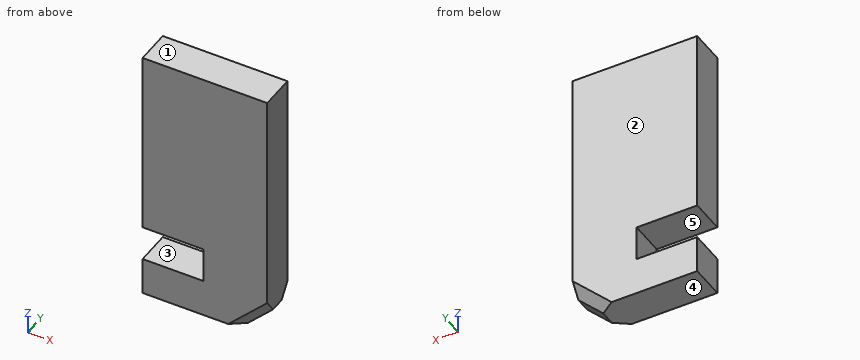
from build123d import *

# Parameters (mm, degrees)
EXTRUDE_1_DEPTH = 14
CHAMFER_1_SIZE  = 4


with BuildPart() as part:
    # 草图1 → 凸台-拉伸1 (new body)
    with BuildSketch(Plane(origin=(0, 0, 0), x_dir=(1, 0, 0), z_dir=(0, 1, 0))):
        Polygon((40, 105), (50, 95), (50, 0), (0, 0), (0, 75.675047551), (24.325372692, 75.675047551), (24.325372692, 89.813954871), (0, 89.813954871), (0, 105), align=None)
    extrude(amount=EXTRUDE_1_DEPTH)

    # 倒角1
    chamfer_1_edges = [part.edges().sort_by_distance(p)[0] for p in [
        (45, 0, -100),
        (45, 14, -100),
    ]]
    chamfer(chamfer_1_edges, length=CHAMFER_1_SIZE)


solid = part.part
Check sheet for the modelled part. Datum: model origin and axes. Units: mm. Face numbers are marked on the shaded views. A direction names the side the tool comes from. Give positions to 0.01 mm unless a question says otherwise; leave off trailing zeros. Order: outer loops, then holes, each group sorted by start corner. A loop starts at its lowest first (then second) coordinate and runs counter-clockwise, first axis right, second up. Notation, with made-up numbers: M 15.5,-40 L 24.5,-40 A24 ccw 24.5,-11 Z; hole C 15.5,88.5 d4. An arc over 180 degrees is marked long. Answer as CSV lines item,"result". Start each with the question number.
Item 1: Cross-section at C-C on x = 44.5. Enter the section's corners in (y, z), plus the area to 3 significant figures.
Item 2: Tool access check on the marked faces 4 and 5. Record the directions out of +Z, -Z, +X, -X, +Y, -Y that give a thin tool (end or side, any length) a straight path to the whole face; none if there is none.
Item 3: Cross-section at A-A on x = 22. Enter the section's corners in (y, z).
Item 4: Thickness scan on line 1 (Z direction, x = 9.5, y = 11.5); line 2 (X direction, y = 11.5, z = -88); line 3 (X direction, y = 0.75, z = -99.5). Record the ranges inside material, lowest first. Write a range as [from, to].
Item 5: Mould release check, pull along Z, two halves, no side actions. Record for the marked faces 1, 2 and 3: +Z half, -Z half, draft (parallel to the pull), parting line (faces both ways), or undercut.
Item 6: Gauge pin test, flat end, axial feed: P1, Ø1.5, axis at x = 19, z = -91, coming from the -Y side. Record the tip position at first contact, or that the pin passes through.
Item 7: Cross-section at D-D on z = -93.5. Enter the section's corners in (x, y), plus the area to 3 significant figures.
Item 8: Cross-section at B-B on y = 5.75. Enter the section's corners in (x, z).
Established:
1,outline,"M 0,-94.84 L 4,-100.5 L 10,-100.5 L 14,-94.84 L 14,0 L 0,0 Z"
1,area,"1,380 mm^2"
2,face 4,"-Z, +X, -X, +Y, -Y"
2,face 5,"-X, +Y, -Y"
3,outline,"M 0,-105 L 14,-105 L 14,-89.81 L 0,-89.81 Z; M 0,-75.68 L 14,-75.68 L 14,0 L 0,0 Z"
4,line 1,"z = [-105, -89.81], [-75.68, 0]"
4,line 2,"x = [24.33, 50]"
4,line 3,"x = [0, 40.9]"
5,face 1,"+Z half"
5,face 2,"draft"
5,face 3,"undercut"
6,P1,"stops at y = 0"
7,outline,"M 0,0 L 45.84,0 L 50,2.94 L 50,11.06 L 45.84,14 L 0,14 Z"
7,area,"688 mm^2"
8,outline,"M 0,-105 L 40,-105 L 50,-95 L 50,0 L 0,0 L 0,-75.68 L 24.33,-75.68 L 24.33,-89.81 L 0,-89.81 Z"
